The model under review builds one solid part; all positions refer to its coordinate system, in mm. Face numbers are marked on the shaded views. Round coordinates to 2 decimals unless told otherwise and drop trailing zeros. Order: outer loops, then holes, each group sorted by start corner. A loop starts at its lowest first (then second) coordinate and runs counter-clockwise, first axis right, second up. Notation, with made-up numbers: (33, 28) -> (62, 28) arc R14 cw to (62, 55) -> close; hole circle Ø10 at (-32.75, 72.25). An arc over 180 degrees is marked (long way). Use a Markdown table: item, result. Add a question column.
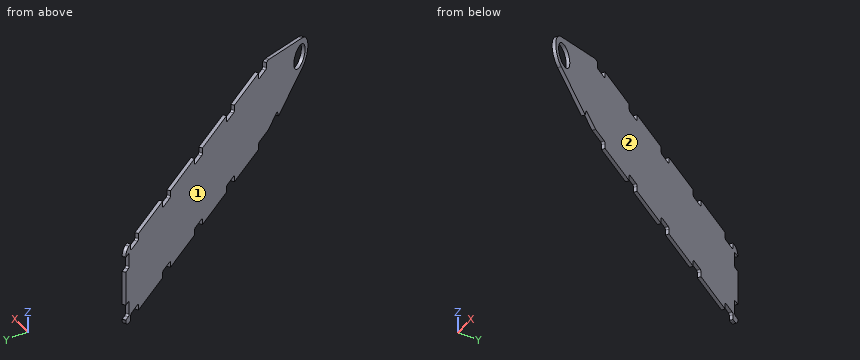
```python
from build123d import *

# Parameters (mm, degrees)
SKETCH1_R           = 42.291
BOSS_EXTRUDE1_DEPTH = 12.7


with BuildPart() as part:
    # Sketch1 → Boss-Extrude1 (new body)
    with BuildSketch(Plane(origin=(106.603890681, 69.014006689, 0), x_dir=(-0.543445635, 0.839444365, 0), z_dir=(0.839444365, 0.543445635, 0))):
        with BuildLine():
            Line((2433.75688, -117.142768), (2433.75688, -136.700768))
            Line((2433.75688, -136.700768), (2445.44088, -136.700768))
            ThreePointArc((2445.44088, -136.700768), (2463.401392242, -129.261280242), (2470.84088, -111.300768))
            Line((2470.84088, -111.300768), (2470.84088, -109.141768))
            Line((2470.84088, -109.141768), (2451.28288, -109.141768))
            ThreePointArc((2451.28288, -109.141768), (2446.792751939, -107.28189606), (2444.93288, -102.791768))
            Line((2444.93288, -102.791768), (2444.93288, -56.309772))
            ThreePointArc((2444.93288, -56.309772), (2446.792751939, -51.819643939), (2451.28288, -49.959772))
            Line((2451.28288, -49.959772), (2470.84088, -49.959772))
            Line((2470.84088, -49.959772), (2470.84088, 81.358228))
            Line((2470.84088, 81.358228), (2451.28288, 81.358228))
            ThreePointArc((2451.28288, 81.358228), (2446.792751939, 83.21809994), (2444.93288, 87.708228))
            Line((2444.93288, 87.708228), (2444.93288, 134.190232))
            ThreePointArc((2444.93288, 134.190232), (2446.792751939, 138.680360061), (2451.28288, 140.540232))
            Line((2451.28288, 140.540232), (2470.84088, 140.540232))
            Line((2470.84088, 140.540232), (2470.84088, 142.699232))
            ThreePointArc((2470.84088, 142.699232), (2463.401392242, 160.659744242), (2445.44088, 168.099232))
            Line((2445.44088, 168.099232), (2433.75688, 168.099232))
            Line((2433.75688, 168.099232), (2433.75688, 148.541232))
            ThreePointArc((2433.75688, 148.541232), (2431.897008061, 144.051103939), (2427.40688, 142.191232))
            Line((2427.40688, 142.191232), (2380.92488, 142.191232))
            ThreePointArc((2380.92488, 142.191232), (2376.434751939, 144.051103939), (2374.57488, 148.541232))
            Line((2374.57488, 148.541232), (2374.57488, 168.099232))
            Line((2374.57488, 168.099232), (2192.45688, 168.099232))
            Line((2192.45688, 168.099232), (2192.45688, 148.541232))
            ThreePointArc((2192.45688, 148.541232), (2190.597008061, 144.051103939), (2186.10688, 142.191232))
            Line((2186.10688, 142.191232), (2139.62488, 142.191232))
            ThreePointArc((2139.62488, 142.191232), (2135.134751939, 144.051103939), (2133.27488, 148.541232))
            Line((2133.27488, 148.541232), (2133.27488, 168.099232))
            Line((2133.27488, 168.099232), (1951.15688, 168.099232))
            Line((1951.15688, 168.099232), (1951.15688, 148.541232))
            ThreePointArc((1951.15688, 148.541232), (1949.297008061, 144.051103939), (1944.80688, 142.191232))
            Line((1944.80688, 142.191232), (1898.32488, 142.191232))
            ThreePointArc((1898.32488, 142.191232), (1893.834751939, 144.051103939), (1891.97488, 148.541232))
            Line((1891.97488, 148.541232), (1891.97488, 168.099232))
            Line((1891.97488, 168.099232), (1709.85688, 168.099232))
            Line((1709.85688, 168.099232), (1709.85688, 148.541232))
            ThreePointArc((1709.85688, 148.541232), (1707.997008061, 144.051103939), (1703.50688, 142.191232))
            Line((1703.50688, 142.191232), (1657.02488, 142.191232))
            ThreePointArc((1657.02488, 142.191232), (1652.534751939, 144.051103939), (1650.67488, 148.541232))
            Line((1650.67488, 148.541232), (1650.67488, 168.099232))
            Line((1650.67488, 168.099232), (1468.55688, 168.099232))
            Line((1468.55688, 168.099232), (1468.55688, 148.541232))
            ThreePointArc((1468.55688, 148.541232), (1466.697008061, 144.051103939), (1462.20688, 142.191232))
            Line((1462.20688, 142.191232), (1415.72488, 142.191232))
            ThreePointArc((1415.72488, 142.191232), (1411.234751939, 144.051103939), (1409.37488, 148.541232))
            Line((1409.37488, 148.541232), (1409.37488, 168.099232))
            Line((1409.37488, 168.099232), (1397.098564625, 168.099232))
            ThreePointArc((1397.098564625, 168.099232), (1392.687900912, 167.713348927), (1388.411252984, 166.567424568))
            Line((1388.411252984, 166.567424568), (1137.847600899, 75.36971342))
            ThreePointArc((1137.847600899, 75.36971342), (1096.06588, 15.699232), (1137.847600899, -43.97124942))
            Line((1137.847600899, -43.97124942), (1317.752937975, -109.451437101))
            Line((1317.752937975, -109.451437101), (1324.442167938, -91.072928824))
            ThreePointArc((1324.442167938, -91.072928824), (1327.725590118, -87.489702286), (1332.58104399, -87.277708592))
            Line((1332.58104399, -87.277708592), (1396.135987148, -110.409816142))
            ThreePointArc((1396.135987148, -110.409816142), (1397.20514913, -110.696297232), (1398.307815058, -110.792768))
            Line((1398.307815058, -110.792768), (1462.20688, -110.792768))
            ThreePointArc((1462.20688, -110.792768), (1466.697008061, -112.652639939), (1468.55688, -117.142768))
            Line((1468.55688, -117.142768), (1468.55688, -136.700768))
            Line((1468.55688, -136.700768), (1650.67488, -136.700768))
            Line((1650.67488, -136.700768), (1650.67488, -117.142768))
            ThreePointArc((1650.67488, -117.142768), (1652.534751939, -112.652639939), (1657.02488, -110.792768))
            Line((1657.02488, -110.792768), (1703.50688, -110.792768))
            ThreePointArc((1703.50688, -110.792768), (1707.997008061, -112.652639939), (1709.85688, -117.142768))
            Line((1709.85688, -117.142768), (1709.85688, -136.700768))
            Line((1709.85688, -136.700768), (1891.97488, -136.700768))
            Line((1891.97488, -136.700768), (1891.97488, -117.142768))
            ThreePointArc((1891.97488, -117.142768), (1893.834751939, -112.652639939), (1898.32488, -110.792768))
            Line((1898.32488, -110.792768), (1944.80688, -110.792768))
            ThreePointArc((1944.80688, -110.792768), (1949.297008061, -112.652639939), (1951.15688, -117.142768))
            Line((1951.15688, -117.142768), (1951.15688, -136.700768))
            Line((1951.15688, -136.700768), (2133.27488, -136.700768))
            Line((2133.27488, -136.700768), (2133.27488, -117.142768))
            ThreePointArc((2133.27488, -117.142768), (2135.134751939, -112.652639939), (2139.62488, -110.792768))
            Line((2139.62488, -110.792768), (2186.10688, -110.792768))
            ThreePointArc((2186.10688, -110.792768), (2190.597008061, -112.652639939), (2192.45688, -117.142768))
            Line((2192.45688, -117.142768), (2192.45688, -136.700768))
            Line((2192.45688, -136.700768), (2374.57488, -136.700768))
            Line((2374.57488, -136.700768), (2374.57488, -117.142768))
            ThreePointArc((2374.57488, -117.142768), (2376.434751939, -112.652639939), (2380.92488, -110.792768))
            Line((2380.92488, -110.792768), (2427.40688, -110.792768))
            ThreePointArc((2427.40688, -110.792768), (2431.897008061, -112.652639939), (2433.75688, -117.142768))
        make_face()
        with Locations(Location((1159.56588, 15.699232, 0), (0, 0, 180))):  # turned: the seam where the file's is
            Circle(SKETCH1_R, mode=Mode.SUBTRACT)
    extrude(amount=-BOSS_EXTRUDE1_DEPTH)


solid = part.part
```
Q1. Mouldability with a two-part tool opening along X and no side actions: class the marked faces 1 and 2 as pulls with the +X half, pulls with the -X half, needs draft (parallel to the pull), parting line crosses it, or undercut.
Q2. Add section B-B (z = -70). Write out the cut boundary in (x, y).
Q3. Wall thickness on line 1 (Y direction, x = -608.5, z = -48); line 2 (X direction, y = 1894, z = 76); line 3 (Y direction, x = -1032, z = -49.5): over which ranges is each line inside the solid? List them lowest first. Write a range as [from, to].
Q4. Add section A-A (x = -1125). Write out the cut boundary in (y, z), then the cut area to 3 significant figures.
Q5. Insertion check: pin 1 (18 mm diameter, centred on x = -1201.5, y = 2077, fed in from -Z); pin 2 (1.5 mm diameter, centred on y = 1738, z = -33, fed in from +X); pin 3 (4 mm diameter, centred on x = -794, z = 78.5, fed in from +Y). Each pin has a flat end and moves straight along its axis. Give the tip position at first contact, or say it passes through.
Report:
| question | item | result |
|---|---|---|
| 1 | face 1 | pulls with the -X half |
| 1 | face 2 | pulls with the +X half |
| 2 | outline | (-1232.75, 2114.5) -> (-561.28, 1077.3) -> (-550.62, 1084.21) -> (-1222.08, 2121.4) -> close |
| 3 | line 1 | y = [1150.24, 1173.61] |
| 3 | line 2 | x = [-1090, -1074.87] |
| 3 | line 3 | y = [1804.41, 1827.78] |
| 4 | outline | (1948.07, -136.7) -> (1971.44, -136.7) -> (1971.44, 168.1) -> (1948.07, 168.1) -> close |
| 4 | area | 7,120 mm² |
| 5 | pin 1 | stops at z = -110.79 |
| 5 | pin 2 | stops at x = -973.39 |
| 5 | pin 3 | stops at y = 1463.24 |
